Work out the finished part from the listing and answer in its coordinate system (mm). A direction names the side the tool comes from. Round coordinates to 2 decimals unless told otherwise and drop trailing zeros. Order: outer loops, then holes, each group sorted by start corner. A loop starts at its lowest first (then second) coordinate and runs counter-clockwise, first axis right, second up. Notation, with made-up numbers: (-34.75, 18) - (16.25, 18) arc R24 cw to (16.25, 52) - close; hole circle Ø6 at (88.25, 21). An arc over 180 degrees is marked (long way). Put each result on its own line as item: value.
```python
from build123d import *

# Parameters (mm, degrees)
BOSS_EXTRUDE1_DEPTH                        = 12.7
SKETCH8_R                                  = 3.3
CUT_EXTRUDE1_DEPTH                         = 12.7
LPATTERN1_COUNT                            = 6
LPATTERN1_PITCH                            = 50
MIRROR1_COPY_1_SKETCH_R                    = 3.3
MIRROR1_COPY_1_DEPTH                       = 12.7
MIRROR1_COPY_2_SKETCH_R                    = 3.3
MIRROR1_COPY_2_DEPTH                       = 12.7
MIRROR1_COPY_3_SKETCH_R                    = 3.3
MIRROR1_COPY_3_DEPTH                       = 12.7
MIRROR1_COPY_4_SKETCH_R                    = 3.3
MIRROR1_COPY_4_DEPTH                       = 12.7
MIRROR1_COPY_5_SKETCH_R                    = 3.3
MIRROR1_COPY_5_DEPTH                       = 12.7
SKETCH14_R                                 = 3.2
CUT_EXTRUDE6_DEPTH                         = 190.436770454
CIRPATTERN1_COUNT                          = 6
FILLET1_R                                  = 2
CUT_EXTRUDE7_REACH                         = 191.437
SKETCH15_R                                 = 5
CUT_EXTRUDE8_REACH                         = 191.437
SKETCH17_R                                 = 5
MIRROR2_AT_THE_SECOND_PLANE_COPY_1_REACH   = 191.437
MIRROR2_AT_THE_SECOND_PLANE_COPY_1_SKETC_R = 5
CUT_EXTRUDE9_REACH                         = 191.437
SKETCH18_W                                 = 38
SKETCH18_H                                 = 25
FILLET3_R                                  = 2


with BuildPart() as part:
    # Sketch2 → Boss-Extrude1 (new body)
    with BuildSketch(Plane(origin=(0, 0, 0), x_dir=(1, 0, 0), z_dir=(0, 1, 0))):
        Polygon((-97.32233047, 150), (97.32233047, 150), (115, 132.32233047), (115, -132.32233047), (97.32233047, -150), (-97.32233047, -150), (-115, -132.32233047), (-115, 132.32233047), align=None)
    extrude(amount=BOSS_EXTRUDE1_DEPTH)

    # Sketch8 → Cut-Extrude1 (cut)
    with BuildSketch(Plane(origin=(0, 12.7, 0), x_dir=(1, 0, 0), z_dir=(0, 1, 0))):
        with Locations(Location((95, -125, 0), (0, 0, 270))):
            Circle(SKETCH8_R)
    cut_extrude1 = extrude(amount=-CUT_EXTRUDE1_DEPTH, mode=Mode.SUBTRACT)

    # LPattern1: Cut-Extrude1 ×6
    with Locations(*[(0, 0, -i * LPATTERN1_PITCH) for i in range(1, LPATTERN1_COUNT)]):
        add(cut_extrude1, mode=Mode.SUBTRACT)

    # Mirror1: Cut-Extrude1 across plane
    add(cut_extrude1.mirror(Plane(origin=(0, 0, 0), x_dir=(0, 0, 1), z_dir=(1, 0, 0))), mode=Mode.SUBTRACT)

    # Mirror1 copy 1 sketch → Mirror1 copy 1 (cut)
    with BuildSketch(Plane(origin=(0, 12.7, -50), x_dir=(-1, 0, 0), z_dir=(0, 1, 0))):
        with Locations((95, 125)):
            Circle(MIRROR1_COPY_1_SKETCH_R)
    extrude(amount=-MIRROR1_COPY_1_DEPTH, mode=Mode.SUBTRACT)

    # Mirror1 copy 2 sketch → Mirror1 copy 2 (cut)
    with BuildSketch(Plane(origin=(0, 12.7, -100), x_dir=(-1, 0, 0), z_dir=(0, 1, 0))):
        with Locations((95, 125)):
            Circle(MIRROR1_COPY_2_SKETCH_R)
    extrude(amount=-MIRROR1_COPY_2_DEPTH, mode=Mode.SUBTRACT)

    # Mirror1 copy 3 sketch → Mirror1 copy 3 (cut)
    with BuildSketch(Plane(origin=(0, 12.7, -150), x_dir=(-1, 0, 0), z_dir=(0, 1, 0))):
        with Locations((95, 125)):
            Circle(MIRROR1_COPY_3_SKETCH_R)
    extrude(amount=-MIRROR1_COPY_3_DEPTH, mode=Mode.SUBTRACT)

    # Mirror1 copy 4 sketch → Mirror1 copy 4 (cut)
    with BuildSketch(Plane(origin=(0, 12.7, -200), x_dir=(-1, 0, 0), z_dir=(0, 1, 0))):
        with Locations((95, 125)):
            Circle(MIRROR1_COPY_4_SKETCH_R)
    extrude(amount=-MIRROR1_COPY_4_DEPTH, mode=Mode.SUBTRACT)

    # Mirror1 copy 5 sketch → Mirror1 copy 5 (cut)
    with BuildSketch(Plane(origin=(0, 12.7, -250), x_dir=(-1, 0, 0), z_dir=(0, 1, 0))):
        with Locations((95, 125)):
            Circle(MIRROR1_COPY_5_SKETCH_R)
    extrude(amount=-MIRROR1_COPY_5_DEPTH, mode=Mode.SUBTRACT)

    # Sketch14 → Cut-Extrude6 (cut, through all)
    with BuildSketch(Plane.XZ):
        with Locations(Location((0, 69.5, 0), (0, 0, 270))):
            Circle(SKETCH14_R)
    cut_extrude6 = extrude(amount=-CUT_EXTRUDE6_DEPTH, mode=Mode.SUBTRACT)

    # CirPattern1: Cut-Extrude6 ×6 about axis
    cirpattern1_axis = Axis((0, 0, -0.032912313), (0, 1, 0))
    for i in range(1, CIRPATTERN1_COUNT):
        add(cut_extrude6.rotate(cirpattern1_axis, i * 360 / CIRPATTERN1_COUNT), mode=Mode.SUBTRACT)

    # Fillet1
    fillet1_edges = [part.edges().sort_by_distance(p)[0] for p in [
        (0, 0, 150),
        (-106.161165235, 0, 141.161165235),
        (-115, 0, 0),
        (-106.161165235, 0, -141.161165235),
        (-106.161165235, 12.7, 141.161165235),
        (-97.32233047, 6.35, -150),
        (97.32233047, 6.35, -150),
        (115, 6.35, -132.32233047),
        (115, 6.35, 132.32233047),
        (97.32233047, 6.35, 150),
        (-97.32233047, 6.35, 150),
        (-115, 6.35, 132.32233047),
        (-115, 6.35, -132.32233047),
        (0, 12.7, 150),
        (106.161165235, 12.7, 141.161165235),
        (115, 12.7, 0),
        (106.161165235, 12.7, -141.161165235),
        (0, 12.7, -150),
        (-106.161165235, 12.7, -141.161165235),
        (0, 0, -150),
        (-115, 12.7, 0),
        (106.161165235, 0, -141.161165235),
        (115, 0, 0),
        (106.161165235, 0, 141.161165235),
    ]]
    fillet(fillet1_edges, radius=FILLET1_R)

    # Sketch15 → Cut-Extrude7 (cut, up to next)
    with BuildSketch(Plane.XZ, mode=Mode.PRIVATE) as cut_extrude7_sk1:
        with Locations(Location((11.64685703, 43.466662183, 0), (0, 0, 270))):
            Circle(SKETCH15_R)
    cut_extrude7_tool1 = extrude(cut_extrude7_sk1.sketch, amount=-CUT_EXTRUDE7_REACH, mode=Mode.PRIVATE) & part.part
    # Sketch15 → Cut-Extrude7 (cut, up to next)
    with BuildSketch(Plane.XZ, mode=Mode.PRIVATE) as cut_extrude7_sk2:
        with Locations(Location((43.466662183, 11.64685703, 0), (0, 0, 270))):
            Circle(SKETCH15_R)
    cut_extrude7_tool2 = extrude(cut_extrude7_sk2.sketch, amount=-CUT_EXTRUDE7_REACH, mode=Mode.PRIVATE) & part.part
    # Sketch15 → Cut-Extrude7 (cut, up to next)
    with BuildSketch(Plane.XZ, mode=Mode.PRIVATE) as cut_extrude7_sk3:
        with Locations(Location((31.819805153, -31.819805153, 0), (0, 0, 270))):
            Circle(SKETCH15_R)
    cut_extrude7_tool3 = extrude(cut_extrude7_sk3.sketch, amount=-CUT_EXTRUDE7_REACH, mode=Mode.PRIVATE) & part.part
    # Sketch15 → Cut-Extrude7 (cut, up to next)
    with BuildSketch(Plane.XZ, mode=Mode.PRIVATE) as cut_extrude7_sk4:
        with Locations(Location((-11.64685703, -43.466662183, 0), (0, 0, 270))):
            Circle(SKETCH15_R)
    cut_extrude7_tool4 = extrude(cut_extrude7_sk4.sketch, amount=-CUT_EXTRUDE7_REACH, mode=Mode.PRIVATE) & part.part
    # Sketch15 → Cut-Extrude7 (cut, up to next)
    with BuildSketch(Plane.XZ, mode=Mode.PRIVATE) as cut_extrude7_sk5:
        with Locations(Location((-43.466662183, -11.64685703, 0), (0, 0, 270))):
            Circle(SKETCH15_R)
    cut_extrude7_tool5 = extrude(cut_extrude7_sk5.sketch, amount=-CUT_EXTRUDE7_REACH, mode=Mode.PRIVATE) & part.part
    # Sketch15 → Cut-Extrude7 (cut, up to next)
    with BuildSketch(Plane.XZ, mode=Mode.PRIVATE) as cut_extrude7_sk6:
        with Locations(Location((-31.819805153, 31.819805153, 0), (0, 0, 270))):
            Circle(SKETCH15_R)
    cut_extrude7_tool6 = extrude(cut_extrude7_sk6.sketch, amount=-CUT_EXTRUDE7_REACH, mode=Mode.PRIVATE) & part.part
    add(cut_extrude7_tool1.solids().sort_by_distance((11.646857, 0, 43.466662))[0], mode=Mode.SUBTRACT)
    add(cut_extrude7_tool2.solids().sort_by_distance((43.466662, 0, 11.646857))[0], mode=Mode.SUBTRACT)
    add(cut_extrude7_tool3.solids().sort_by_distance((31.819805, 0, -31.819805))[0], mode=Mode.SUBTRACT)
    add(cut_extrude7_tool4.solids().sort_by_distance((-11.646857, 0, -43.466662))[0], mode=Mode.SUBTRACT)
    add(cut_extrude7_tool5.solids().sort_by_distance((-43.466662, 0, -11.646857))[0], mode=Mode.SUBTRACT)
    add(cut_extrude7_tool6.solids().sort_by_distance((-31.819805, 0, 31.819805))[0], mode=Mode.SUBTRACT)

    # Sketch17 → Cut-Extrude8 (cut, up to next)
    with BuildSketch(Plane.XZ, mode=Mode.PRIVATE) as cut_extrude8_sk1:
        with Locations(Location((-63, 10.5, 0), (0, 0, 270))):
            Circle(SKETCH17_R)
    cut_extrude8_tool1 = extrude(cut_extrude8_sk1.sketch, amount=-CUT_EXTRUDE8_REACH, mode=Mode.PRIVATE) & part.part
    cut_extrude8 = cut_extrude8_tool1.solids().sort_by_distance((-63, 0, 10.5))[0]
    add(cut_extrude8, mode=Mode.SUBTRACT)

    # Mirror2: Cut-Extrude8 across plane
    add(cut_extrude8.mirror(Plane.XY), mode=Mode.SUBTRACT)

    # Mirror2 at the second plane: Cut-Extrude8 across plane
    add(cut_extrude8.mirror(Plane(origin=(0, 0, 0), x_dir=(0, 0, 1), z_dir=(1, 0, 0))), mode=Mode.SUBTRACT)

    # Mirror2 at the second plane copy 1 sketc → Mirror2 at the second plane copy 1 (cut, up to next)
    with BuildSketch(Plane(origin=(0, 0, 0), x_dir=(-1, 0, 0), z_dir=(0, -1, 0)), mode=Mode.PRIVATE) as mirror2_at_the_second_plane_copy_1_sk1:
        with Locations(Location((-63, 10.5, 0), (0, 0, 270))):
            Circle(MIRROR2_AT_THE_SECOND_PLANE_COPY_1_SKETC_R)
    mirror2_at_the_second_plane_copy_1_tool1 = extrude(mirror2_at_the_second_plane_copy_1_sk1.sketch, amount=-MIRROR2_AT_THE_SECOND_PLANE_COPY_1_REACH, mode=Mode.PRIVATE) & part.part
    add(mirror2_at_the_second_plane_copy_1_tool1.solids().sort_by_distance((63, 0, -10.5))[0], mode=Mode.SUBTRACT)

    # Sketch18 → Cut-Extrude9 (cut, up to next)
    with BuildSketch(Plane.XZ, mode=Mode.PRIVATE) as cut_extrude9_sk1:
        with Locations((0, 43.08)):
            Rectangle(SKETCH18_W, SKETCH18_H)
    cut_extrude9_tool1 = extrude(cut_extrude9_sk1.sketch, amount=-CUT_EXTRUDE9_REACH, mode=Mode.PRIVATE) & part.part
    add(cut_extrude9_tool1.solids().sort_by_distance((0, 0, 43.08))[0], mode=Mode.SUBTRACT)

    # Fillet3
    fillet3_edges = [part.edges().sort_by_distance(p)[0] for p in [
        (-19, 6.35, 30.58),
        (-19, 6.35, 55.58),
        (19, 6.35, 55.58),
        (19, 6.35, 30.58),
        (-19, 0, 43.08),
        (0, 0, 30.58),
        (19, 0, 43.08),
        (0, 0, 55.58),
        (0, 12.7, 30.58),
        (-19, 12.7, 43.08),
        (0, 12.7, 55.58),
        (19, 12.7, 43.08),
    ]]
    fillet(fillet3_edges, radius=FILLET3_R)


solid = part.part
```
1) A cutting plane is placed at D-D on y = 6. Give the number of separate pieces and of enclosed holes in the cut face, then the cut area to 3 significant figures.
Findings below:
separate pieces: 1
enclosed holes: 28
area: 66,100 mm2
2) For a pull along Z with two mould halves and no side action, classify faces 3 (the cylindrical face through (-97.23, 6.44, 122.57)), 4 (the flat face through (-106.277, 6.289, -141.046)), 5 (the flat face through (115, 6, -2)), 6 (the cylindrical face through (-91.7, 6.4, -24.9)) as pulls with the +Z half, pulls with the -Z half, needs draft (parallel to the pull), parting line crosses it, or undercut.
Findings below:
face 3: undercut
face 4: pulls with the -Z half
face 5: needs draft
face 6: undercut
3) Given pin 1 Ø6 at (x, z) = (79.5, -94.5) entering from -Y; pin 2 Ø5.5 at (x, z) = (95, 25) entering from +Y, each flat-ended and moving along its own axis, determine where each tip first touches the part or whether it passes through.
Findings below:
pin 1: stops at y = 0
pin 2: passes through
4) For faces 1 (the flat face through (-19, 6, 43)), 2 (the flat face through (106.046, 6.289, -141.277)), determine the directions among +Z, -Z, +X, -X, +Y, -Y from which every point of the face is accessible in a straight line to the end or side of a thin tool.
Findings below:
face 1: +Y, -Y
face 2: -Z, +X, +Y, -Y
5) A cutting plane is placed at A-A on x = 0. Write down the section's boundary in (y, z).
Findings below:
outline: (0, -148) arc R2 ccw to (2, -150) - (10.7, -150) arc R2 ccw to (12.7, -148) - (12.7, -72.77) - (0, -72.77) - close; (0, -66.37) - (12.7, -66.37) - (12.7, 28.58) arc R2 ccw to (10.7, 30.58) - (2, 30.58) arc R2 ccw to (0, 28.58) - close; (0, 57.58) arc R2 ccw to (2, 55.58) - (10.7, 55.58) arc R2 ccw to (12.7, 57.58) - (12.7, 66.3) - (0, 66.3) - close; (0, 72.7) - (12.7, 72.7) - (12.7, 148) arc R2 ccw to (10.7, 150) - (2, 150) arc R2 ccw to (0, 148) - close
6) A cutting plane is placed at C-C on z = -44.5. Write down the section's boundary in (x, y).
Findings below:
outline: (-115, 2) arc R2 ccw to (-113, 0) - (-16.54, 0) - (-16.54, 12.7) - (-113, 12.7) arc R2 ccw to (-115, 10.7) - close; (-6.75, 0) - (113, 0) arc R2 ccw to (115, 2) - (115, 10.7) arc R2 ccw to (113, 12.7) - (-6.75, 12.7) - close
7) Straight lines are drawn through the part: L1, parallel to X at y = 4, z = 24.5; L2, parallel to Z at x = 12.5, y = 8; L3, parallel to X at y = 3, z = -10.5. For each, find the intervals that lie inside material, in ascending order. Write a range as from..to.
Findings below:
L1: x = -115..-98.26, -91.74..91.74, 98.26..115
L2: z = -150..30.58, 55.58..150
L3: x = -115..-68, -58..-48.33, -38.6..58, 68..115
8) A cutting plane is placed at B-B on z = 10.5. Write down the section's boundary in (x, y), then the cut area to 3 significant figures.
Findings below:
outline: (-115, 2) arc R2 ccw to (-113, 0) - (-68, 0) - (-68, 12.7) - (-113, 12.7) arc R2 ccw to (-115, 10.7) - close; (-58, 0) - (38.6, 0) - (38.6, 12.7) - (-58, 12.7) - close; (48.33, 0) - (58, 0) - (58, 12.7) - (48.33, 12.7) - close; (68, 0) - (113, 0) arc R2 ccw to (115, 2) - (115, 10.7) arc R2 ccw to (113, 12.7) - (68, 12.7) - close
area: 2,540 mm2
